```python
from build123d import *

# Parameters (mm, degrees)
SKETCH1_R           = 21
BOSS_EXTRUDE1_DEPTH = 50
SKETCH2_W           = 20
SKETCH2_H           = 22
BOSS_EXTRUDE2_DEPTH = 2.5
FILLET1_R           = 5
FILLET2_R           = 5
SKETCH3_R           = 4
CUT_EXTRUDE1_DEPTH  = 24.5


with BuildPart() as part:
    # Sketch1 → Boss-Extrude1 (new body)
    with BuildSketch(Plane.XY):
        Circle(SKETCH1_R)
    extrude(amount=BOSS_EXTRUDE1_DEPTH)

    # Sketch2 → Boss-Extrude2 (add, symmetric)
    with BuildSketch(Plane(origin=(0, 0, 0), x_dir=(0, 0, -1), z_dir=(1, 0, 0))):
        with Locations((-60, 0)):
            Rectangle(SKETCH2_W, SKETCH2_H)
    extrude(amount=BOSS_EXTRUDE2_DEPTH, both=True)

    # Fillet1
    fillet1_edges = [part.edges().sort_by_distance(p)[0] for p in [
        (-2.5, 0, 50),
        (0, -11, 50),
        (0, 11, 50),
        (2.5, 0, 50),
    ]]
    fillet(fillet1_edges, radius=FILLET1_R)

    # Fillet2
    fillet2_edges = [part.edges().sort_by_distance(p)[0] for p in [
        (0, 11, 70),
        (0, -11, 70),
    ]]
    fillet(fillet2_edges, radius=FILLET2_R)

    # Sketch3 → Cut-Extrude1 (cut, through all)
    with BuildSketch(Plane(origin=(2.5, 0, 0), x_dir=(0, 0, -1), z_dir=(1, 0, 0))):
        with Locations((-62.5, 0)):
            Circle(SKETCH3_R)
    extrude(amount=-CUT_EXTRUDE1_DEPTH, mode=Mode.SUBTRACT)


solid = part.part
```
Geometry: final body of the model. Coordinates: model frame, mm. A direction names the side the tool comes from. Round coordinates to 2 decimals unless told otherwise and drop trailing zeros. Write each loop counter-clockwise with the first axis right and the second up, starting at its lowest first coordinate (ties: lowest second). Pieces come first, ordered by that corner, then holes. Notation, with made-up numbers: (35, 26.25) -> (65, 26.25) arc R11 cw to (65, 31.25) -> close; hole circle Ø3 at (58, -10.75). An arc over 180 degrees is marked (long way). Return JSON: item names as keys, results as strings.
Q1. Section A-A on y = 0. Return the cut outline in (x, z).
From the geometry:
{"outline": "(-21, 0) -> (21, 0) -> (21, 50) -> (7.5, 50) arc R5 cw to (2.5, 55) -> (2.5, 58.5) -> (-2.5, 58.5) -> (-2.5, 55) arc R5 cw to (-7.5, 50) -> (-21, 50) -> close; (-2.5, 66.5) -> (2.5, 66.5) -> (2.5, 70) -> (-2.5, 70) -> close"}
Q2. First-contact query: pin 1 Ø7.5 at (y, z) = (1, 62) entering from +X; pin 2 Ø12 at (x, z) = (-1, 12) entering from -Y; pin 3 Ø5.5 at (x, z) = (0, 57.5) entering from -Y. Flat tips, straight axial feed; report the tip coordinate or a pass-through.
From the geometry:
{"pin 1": "x = 2.5", "pin 2": "y = -21", "pin 3": "y = -11.01"}
Q3. Ray query, line 1 (Y direction, x = 1.15, z = 62.5); line 2 (Z direction, x = -12, y = -8.5); line 3 (X direction, y = 8, z = 61.5). Return the intervals inside material, ascending.
From the geometry:
{"line 1": "-11 to -4, 4 to 11", "line 2": "0 to 50", "line 3": "-2.5 to 2.5"}
Q4. Set-up query: faces 1 (the flat face through (0, 11, 60)), 2 (the flat face through (-2.5, 3, 59)), 3 (the flat face through (0, 0, 70)), 4 (the flat face through (0, -11, 60)), 5 (the flat face through (2.5, 3, 59)). Return all of +Z, -Z, +X, -X, +Y, -Y with unobstructed straight access to the full face (end or side cutting, diameter ignored); none if empty.
From the geometry:
{"face 1": "+Z, +X, -X, +Y", "face 2": "+Z, -X, +Y, -Y", "face 3": "+Z, +X, -X, +Y, -Y", "face 4": "+Z, +X, -X, -Y", "face 5": "+Z, +X, +Y, -Y"}
Q5. Section C-C on z = 64. Return the cut outline in (x, y), and give its area (3 significant figures).
From the geometry:
{"outline": "(-2.5, -11) -> (2.5, -11) -> (2.5, -3.71) -> (-2.5, -3.71) -> close; (-2.5, 3.71) -> (2.5, 3.71) -> (2.5, 11) -> (-2.5, 11) -> close", "area": "72.9 mm2"}
Q6. Section D-D on y = 9. Return the cut outline in (x, z), and give its area (3 significant figures).
From the geometry:
{"outline": "(-18.97, 0) -> (18.97, 0) -> (18.97, 50) -> (7.5, 50) arc R5 cw to (2.5, 55) -> (2.5, 69) -> (-2.5, 69) -> (-2.5, 55) arc R5 cw to (-7.5, 50) -> (-18.97, 50) -> close", "area": "2,000 mm2"}
Q7. Section B-B on x = 0. Return the cut outline in (y, z).
From the geometry:
{"outline": "(-21, 0) -> (21, 0) -> (21, 50) -> (16, 50) arc R5 cw to (11, 55) -> (11, 65) arc R5 ccw to (6, 70) -> (-6, 70) arc R5 ccw to (-11, 65) -> (-11, 55) arc R5 cw to (-16, 50) -> (-21, 50) -> close; hole circle Ø8 at (0, 62.5)"}
